Build history of the part. All positions in model axes, mm. A direction names the side the tool comes from. Give positions to 0.01 mm unless a question says otherwise; leave off trailing zeros. Loops run counter-clockwise (first coordinate to the right, second up) from the corner with the lowest first, then second, coordinate; pieces in that order, holes last.
1) 3-axis set-ups, long thin cutter, end or side, ignore diameter. For faces 4 (the flat face through (5.5, 4, -12)), 5 (the cylindrical face through (2.215, 3.125, 11.521)), 6 (the flat face through (0, 3, 10)): which of +Z, -Z, +X, -X, +Y, -Y reach the whole face in a straight line?
2) Band-saw the part on C-C on y = 4.5. List the corners of the cut face in (x, z), then the cut area to 3 significant figures.
3) Band-saw the part on A-A on x = 1.5. List the corners of the cut face in (y, z).
4) Band-saw the part on B-B on x = 4.5. List the corners of the cut face in (y, z), then the cut area to 3 significant figures.
5) Wall check: line 1 (Z direction, x = 4.5, y = 4); line 2 (Y direction, x = 1.5, z = 11.8); line 3 (X direction, y = 7.5, z = -5). Give the ranges that are in metal, low to high.
6) Band-saw the part on D-D on y = 7.5. List the corners of the cut face in (x, z), then the cut area to 3 significant figures.
7) Flat gauge pins, fed straight in: P1, Ø2, axis at x = -1, z = 2.5, coming from the -Y side; P2, Ø2, axis at y = 3.5, z = -19.5, coming from the -X side; P3, Ø4.5, axis at y = 4.5, z = 1.5, coming from the +X side; P4, Ø4, axis at y = 7, z = -21.5, coming from the +X side. Where does each tip first touch, or does it go through?
8) Two-plate mould, pull along Z, no slides. Class faces 1 (the flat face through (0.08, 5.44, 13)), 2 (the flat face through (-5.5, 4, 0)), 3 (the flat face through (-3.156, 4, 0)): +Z half, -Z half, draft (parallel to the pull), parting line (faces both ways), or undercut.
```python
from build123d import *

# Parameters (mm, degrees)
BOSS_EXTRUDE1_DEPTH = 9
SKETCH2_R           = 1.55
CUT_EXTRUDE1_DEPTH  = 10


with BuildPart() as part:
    # Sketch1 → Boss-Extrude1 (new body)
    with BuildSketch(Plane(origin=(0, 0, 0), x_dir=(1, 0, 0), z_dir=(0, 1, 0))):
        with BuildLine():
            Line((5.5, 14.254033308), (5.5, 10))
            Line((5.5, 10), (-3.155943876, 10))
            Line((-3.155943876, 10), (-3.155943876, -10))
            Line((-3.155943876, -10), (5.5, -10))
            Line((5.5, -10), (5.5, -13))
            Line((5.5, -13), (-5.5, -13))
            Line((-5.5, -13), (-5.5, 14.062746067))
            ThreePointArc((-5.5, 14.062746067), (-8.315661291, 19.904731936), (-7.680431732, 26.358663359))
            Line((-7.680431732, 26.358663359), (-4.122387432, 24.428828902))
            ThreePointArc((-4.122387432, 24.428828902), (-2.312437222, 16.503130569), (5.5, 14.254033308))
        make_face()
    extrude(amount=BOSS_EXTRUDE1_DEPTH)

    # Sketch2 → Cut-Extrude1 (cut)
    with BuildSketch(Plane.XY.offset(13)):
        with Locations((1.5, 4.5)):
            Circle(SKETCH2_R)
    extrude(amount=-CUT_EXTRUDE1_DEPTH, mode=Mode.SUBTRACT)


solid = part.part
```
Findings below:
1. face 4: +Z, -Z, +X, +Y, -Y
1. face 5: +Z
1. face 6: +X, +Y, -Y
2. outline: (-7.68, -26.36) - (-4.12, -24.43) arc R8 cw to (5.5, -14.25) - (5.5, -10) - (-3.16, -10) - (-3.16, 10) - (-0.05, 10) - (-0.05, 13) - (-5.5, 13) - (-5.5, -14.06) arc R12 ccw to start; (3.05, 10) - (5.5, 10) - (5.5, 13) - (3.05, 13) - close
2. area: 167 mm2
3. outline: (0, -14.25) - (9, -14.25) - (9, -10) - (0, -10) - close; (0, 10) - (2.95, 10) - (2.95, 13) - (0, 13) - close; (6.05, 10) - (9, 10) - (9, 13) - (6.05, 13) - close
4. outline: (0, -14.06) - (9, -14.06) - (9, -10) - (0, -10) - close; (0, 10) - (9, 10) - (9, 13) - (0, 13) - close
4. area: 63.6 mm2
5. line 1: z = -14.06 to -10, 10 to 13
5. line 2: y = 0 to 2.95, 6.05 to 9
5. line 3: x = -5.5 to -3.16
6. outline: (-7.68, -26.36) - (-4.12, -24.43) arc R8 cw to (5.5, -14.25) - (5.5, -10) - (-3.16, -10) - (-3.16, 10) - (5.5, 10) - (5.5, 13) - (-5.5, 13) - (-5.5, -14.06) arc R12 ccw to start
6. area: 176 mm2
7. P1: passes through
7. P2: stops at x = -8.41
7. P3: stops at x = -3.16
7. P4: stops at x = -4.1
8. face 1: +Z half
8. face 2: draft
8. face 3: undercut
